Verification items for the finished model (mm, model axes). A direction names the side the tool comes from. Round coordinates to 2 decimals unless told otherwise and drop trailing zeros. Order: outer loops, then holes, each group sorted by start corner. A loop starts at its lowest first (then second) coordinate and runs counter-clockwise, first axis right, second up. Notation, with made-up numbers: (-5.75, -37.75) -> (21.25, -37.75) arc R9 ccw to (21.25, -31.75) -> close; hole circle Ø6 at (40, 35.5). An arc over 180 degrees is marked (long way). Return JSON: item names as keys, results as strings. Group by question number.
1) Section check C-C on y = -47. Enter the section's corners in (x, z).
2) Draft check along X on faces 6 (the flat face through (114.3, -25, 19)), 7 (the flat face through (56, -32, 0)), 8 (the flat face through (82.55, -13, 38)). Enter one of: pulls with the +X half, pulls with the -X half, needs draft (parallel to the pull), parting line crosses it, or undercut.
3) Scan lines: L1, parallel to X at y = -13, z = 43.5; L2, parallel to Y at x = 13.5, z = 18.5; L3, parallel to Z at x = 25.5, y = -34. Record each from-to range of solid material in increasing order.
4) Depth check by flat-ended pin: pin 1 (14 mm diameter, centred on x = 7.5, y = -29, fed in from +Z); pin 2 (3 mm diameter, centred on x = 49.5, y = -48.5, fed in from +Z); pin 3 (12 mm diameter, centred on y = -8, z = 44.5, fed in from -X); pin 4 (10 mm diameter, centred on y = -33, z = 43, fed in from +X). Enter the tip coordinate at first touch or a pass-through.
5) Section check D-D on y = -57.5. Enter the section's corners in (x, z), plus the area to 3 significant figures.
6) Tool access check on faces 1 (the flat face through (107, -25, 37.766)), 2 (the flat face through (19.05, -9, 44)), 3 (the flat face through (56, -50.8, 20)), 4 (the flat face through (12.7, -35, 31)), 5 (the flat face through (0, -25, 19)). Record the directions out of +Z, -Z, +X, -X, +Y, -Y that give a thin tool (end or side, any length) a straight path to the whole face; none if there is none.
7) Section check B-B on x = 23. Enter the section's corners in (y, z).
8) Section check A-A on z = 36. Enter the section's corners in (x, y).
```python
from build123d import *

# Parameters (mm, degrees)
F0_W      = 63.5
F0_H      = 12.7
F1_DEPTH  = 114.3
F2_W      = 50.8
F2_H      = 12.7
F3_DEPTH  = 114.3
F6_W      = 12.7
F6_H      = 12.7
F7_DEPTH  = 50.8
F8_W      = 12.7
F8_H      = 12.7
F9_DEPTH  = 50.8
F10_W     = 6.35
F10_H     = 12.7
F11_DEPTH = 19.05
F12_DEPTH = 19.05
F13_W     = 50.8
F13_H     = 6.35
F14_DEPTH = 25.4


with BuildPart() as f1:
    # F0 (on Right) → F1 (new body)
    with BuildSketch(Plane.YZ):
        with Locations((-31.75, 6.35)):
            Rectangle(F0_W, F0_H)
    extrude(amount=F1_DEPTH)

    # F2 (on Right) → F3 (join)
    with BuildSketch(Plane.YZ):
        with Locations((-25.4, 18.7161865272)):
            Rectangle(F2_W, F2_H)
    extrude(amount=F3_DEPTH)

    # F6 (on offset) → F7 (join)
    with BuildSketch(Plane.XZ.offset(50.8)):
        with Locations((6.35, 31.2356372522)):
            Rectangle(F6_W, F6_H)
    extrude(amount=-F7_DEPTH)

    # F8 (on face) → F9 (join)
    with BuildSketch(Plane.XZ.offset(50.8)):
        with Locations((107.95, 31.4161865272)):
            Rectangle(F8_W, F8_H)
    extrude(amount=-F9_DEPTH)

    # F10 (on face) → F11 (join)
    with BuildSketch(Plane(origin=(0, 0, 0), x_dir=(-1, 0, 0), z_dir=(0, 1, 0))):
        with Locations((-98.425, 31.4161865272)):
            Rectangle(F10_W, F10_H)
        with Locations((-15.875, 31.4161865272)):
            Rectangle(F10_W, F10_H)
    extrude(amount=-F11_DEPTH)

    # F10 (on face) → F12 (join)
    with BuildSketch(Plane(origin=(0, 0, 0), x_dir=(-1, 0, 0), z_dir=(0, 1, 0))):
        with Locations((-98.425, 31.4161865272)):
            Rectangle(F10_W, F10_H)
        with Locations((-15.875, 31.4161865272)):
            Rectangle(F10_W, F10_H)
    extrude(amount=-F12_DEPTH)

    # F13 (on face) → F14 (join)
    with BuildSketch(Plane.XY.offset(25.0661865272)):
        Polygon((31.75, 0), (19.05, 0), (19.05, -19.05), (31.75, -19.05), (31.75, -6.35), align=None)
        with Locations((57.15, -3.175)):
            Rectangle(F13_W, F13_H)
        Polygon((95.25, 0), (82.55, 0), (82.55, -6.35), (82.55, -19.05), (95.25, -19.05), align=None)
    extrude(amount=F14_DEPTH)


solid = f1.part
```
Check result:
{
 "1": {"outline": "(0, 0) -> (114.3, 0) -> (114.3, 37.77) -> (101.6, 37.77) -> (101.6, 25.07) -> (12.7, 25.07) -> (12.7, 37.59) -> (0, 37.59) -> close"},
 "2": {"face 6": "pulls with the +X half", "face 7": "needs draft", "face 8": "undercut"},
 "3": {"L1": "19.05 to 31.75, 82.55 to 95.25", "L2": "-50.8 to 0", "L3": "0 to 25.07"},
 "4": {"pin 1": "z = 37.59", "pin 2": "z = 25.07", "pin 3": "x = 19.05", "pin 4": "through"},
 "5": {"outline": "(0, 0) -> (114.3, 0) -> (114.3, 12.7) -> (0, 12.7) -> close", "area": "1,450 mm^2"},
 "6": {"face 1": "+Z, +X, +Y, -Y", "face 2": "+Z, -X, +Y, -Y", "face 3": "+Z, +X, -X, -Y", "face 4": "+Z, -Y", "face 5": "+Z, -Z, -X, +Y, -Y"},
 "7": {"outline": "(-63.5, 0) -> (0, 0) -> (0, 50.47) -> (-19.05, 50.47) -> (-19.05, 25.07) -> (-50.8, 25.07) -> (-50.8, 12.7) -> (-63.5, 12.7) -> close"},
 "8": {"outline": "(0, -50.8) -> (12.7, -50.8) -> (12.7, -19.05) -> (31.75, -19.05) -> (31.75, -6.35) -> (82.55, -6.35) -> (82.55, -19.05) -> (101.6, -19.05) -> (101.6, -50.8) -> (114.3, -50.8) -> (114.3, 0) -> (0, 0) -> close"}
}
